The listing builds one solid part. Answer for the finished solid, in the listing's coordinates (mm). A direction names the side the tool comes from. Coordinates: 2 decimals unless noted, no trailing zeros. Write each loop counter-clockwise with the first axis right and the second up, starting at its lowest first coordinate (ties: lowest second). Pieces come first, ordered by that corner, then holes.
from build123d import *

# Parameters (mm, degrees)
SKETCH_1_W               = 170
SKETCH_1_H               = 90
SKETCH_1_W_2             = 158
SKETCH_1_H_2             = 78
EXTRUDE_1_DEPTH          = 8
SKETCH_2_R               = 2
CUT_EXTRUDE_1_DEPTH      = 177.036927944
SKETCH_3_R               = 2
CUT_EXTRUDE_2_DEPTH      = 125.05240828
CUT_EXTRUDE_3_DEPTH      = 97.509066932
CUT_EXTRUDE_3_DEPTH_BACK = 97.509066932
SKETCH_4_R               = 1.6
EXTRUDE_2_DEPTH          = 8
FILLET_2_R               = 3
FILLET_3_R               = 2


with BuildPart() as part:
    # 草图1 → 凸台-拉伸1 (new body)
    with BuildSketch(Plane.XY):
        Rectangle(SKETCH_1_W, SKETCH_1_H)
        Rectangle(SKETCH_1_W_2, SKETCH_1_H_2, mode=Mode.SUBTRACT)
    extrude(amount=EXTRUDE_1_DEPTH)

    # 草图2 → 切除-拉伸1 (cut, through all)
    with BuildSketch(Plane.ZY.offset(85)):
        with Locations((4, 20)):
            Circle(SKETCH_2_R)
        with Locations((4, -35)):
            Circle(SKETCH_2_R)
    extrude(amount=-CUT_EXTRUDE_1_DEPTH, mode=Mode.SUBTRACT)

    # 草图3 → 切除-拉伸2 (cut, through all)
    with BuildSketch(Plane(origin=(0, 45, 0), x_dir=(1, 0, 0), z_dir=(0, 1, 0))):
        with Locations(Location((-60, -4, 0), (0, 0, 270))):
            Circle(SKETCH_3_R)
        with Locations(Location((60, -4, 0), (0, 0, 270))):
            Circle(SKETCH_3_R)
    extrude(amount=-CUT_EXTRUDE_2_DEPTH, mode=Mode.SUBTRACT)

    # 草图4 → 切除-拉伸3 (cut, two sides: drawn at the far end of the back side and taken through both)
    with BuildSketch(Plane(origin=(0, 0, 0), x_dir=(-1, 0, 0), z_dir=(0, 0, -1)).offset(-CUT_EXTRUDE_3_DEPTH_BACK)):
        with Locations((-82, 30)):
            Circle(SKETCH_4_R)
        with Locations((-82, -30)):
            Circle(SKETCH_4_R)
        with Locations((82, 30)):
            Circle(SKETCH_4_R)
        with Locations((82, -30)):
            Circle(SKETCH_4_R)
        with Locations((-50, 42)):
            Circle(SKETCH_4_R)
        with Locations((50, 42)):
            Circle(SKETCH_4_R)
        with Locations((-50, -42)):
            Circle(SKETCH_4_R)
        with Locations((50, -42)):
            Circle(SKETCH_4_R)
    extrude(amount=CUT_EXTRUDE_3_DEPTH + CUT_EXTRUDE_3_DEPTH_BACK, mode=Mode.SUBTRACT)

    # 草图5 → 凸台-拉伸2 (add)
    with BuildSketch(Plane(origin=(0, 0, 0), x_dir=(-1, 0, 0), z_dir=(0, 0, -1))):
        Polygon((-53.710567135, 39), (-25.320888862, -39), (-20, -39), (-48.389678273, 39), align=None)
        Polygon((53.710567135, 39), (48.389678273, 39), (20, -39), (25.320888862, -39), align=None)
    extrude(amount=-EXTRUDE_2_DEPTH)

    # 圆角2
    fillet_2_edges = [part.edges().sort_by_distance(p)[0] for p in [
        (25.320888862, -39, 4),
        (20, -39, 4),
        (48.389678273, 39, 4),
        (-48.389678273, 39, 4),
        (-20, -39, 4),
        (-25.320888862, -39, 4),
        (79, 39, 4),
        (-79, 39, 4),
    ]]
    fillet(fillet_2_edges, radius=FILLET_2_R)

    # 圆角3
    fillet_3_edges = [part.edges().sort_by_distance(p)[0] for p in [
        (53.710567135, 39, 4),
        (-53.710567135, 39, 4),
    ]]
    fillet(fillet_3_edges, radius=FILLET_3_R)


solid = part.part
Q1. The part is cut by section B-B, the plane y = 42. Write down the section's boundary in (x, z), then the cut area to 3 significant figures.
Answers below:
outline: (-85, 0) - (-51.6, 0) - (-51.6, 8) - (-85, 8) - close; (-48.4, 0) - (48.4, 0) - (48.4, 8) - (-48.4, 8) - close; (51.6, 0) - (85, 0) - (85, 8) - (51.6, 8) - close; hole circle Ø4 at (-60, 4); hole circle Ø4 at (60, 4)
area: 1,280 mm2
Q2. Which of the six approach directions +Z, -Z, +X, -X, +Y, -Y give full straight-line access (tool end or side, diameter ignored) to faces 4 (the face through (-82, 22, 4)), 5 (the face through (82, -37, 4)), 6 (the face through (-1, 39, 4))?
Answers below:
face 4: -X
face 5: +X
face 6: +Z, -Z
Q3. The part is cut by section C-C, the plane x = -60. Write down the section's boundary in (y, z), then the cut area to 3 significant figures.
Answers below:
outline: (-45, 0) - (-39, 0) - (-39, 2) - (-45, 2) - close; (-45, 6) - (-39, 6) - (-39, 8) - (-45, 8) - close; (39, 0) - (45, 0) - (45, 2) - (39, 2) - close; (39, 6) - (45, 6) - (45, 8) - (39, 8) - close
area: 48.0 mm2
Q4. Determine the mould class of faces 1 (the face through (46.54, 37.75, 4.06)), 2 (the face through (-1, 45, 4)), 3 (the face through (85, -1, 4)) for opening direction X: released by +X, released by -X, zero draft, split by the parting line, or undercut.
Answers below:
face 1: undercut
face 2: zero draft
face 3: released by +X
Q5. Given pin 1 (2.5 mm diameter, centred on y = -35, z = 4, fed in from +X); pin 2 (3.5 mm diameter, centred on y = -35, z = 4, fed in from +X); pin 3 (3 mm diameter, centred on y = 20, z = 4, fed in from -X), each flat-ended and moving along its own axis, determine where each tip first touches the part or whether it passes through.
Answers below:
pin 1: stops at x = 27.23
pin 2: stops at x = 27.41
pin 3: stops at x = -47.34
Q6. Find the intervals of material crossed by probe 1 along Y at (x, z) = (-75, 5); probe 2 along X at (y, z) = (27, 2.25); probe 3 along Y at (x, z) = (82, 3.5), in increasing order.
Answers below:
probe 1: y = -45 to -39, 39 to 45
probe 2: x = -85 to -79, -49.34 to -44.02, 44.02 to 49.34, 79 to 85
probe 3: y = -45 to -36.94, -33.06 to -31.6, -28.4 to 18.06, 21.94 to 28.4, 31.6 to 45
Q7. The part is cut by section A-A, the plane x = 82. Write down the section's boundary in (y, z).
Answers below:
outline: (-45, 0) - (-31.6, 0) - (-31.6, 8) - (-45, 8) - close; (-28.4, 0) - (28.4, 0) - (28.4, 8) - (-28.4, 8) - close; (31.6, 0) - (45, 0) - (45, 8) - (31.6, 8) - close; hole circle Ø4 at (-35, 4); hole circle Ø4 at (20, 4)
Q8. The part is cut by section D-D, the plane z = 4. State how many separate pieces and enclosed holes the cut face has, then the cut area to 3 significant figures.
Answers below:
separate pieces: 7
enclosed holes: 9
area: 3,570 mm2
